Geometry check sheet. Reference: the model listing, model coordinates, mm. Face numbers are marked on the shaded views. Coordinates: 2 decimals unless noted, no trailing zeros. Loops run counter-clockwise (first coordinate to the right, second up) from the corner with the lowest first, then second, coordinate; pieces in that order, holes last.
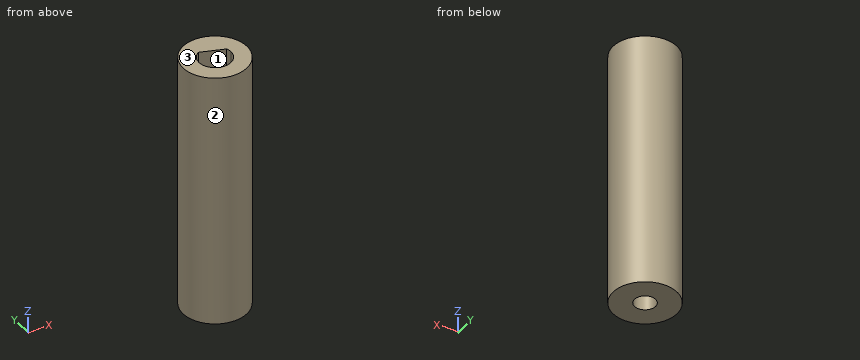
from build123d import *

# Parameters (mm, degrees)
F0_R     = 5
F1_DEPTH = 40
F3_DEPTH = 24
F4_R     = 1.65
F5_DEPTH = 25.4


with BuildPart() as f1:
    # F0 (on Top) → F1 (new body)
    with BuildSketch(Plane.XY):
        Circle(F0_R)
    extrude(amount=F1_DEPTH)

    # F2 (on face) → F3 (cut)
    with BuildSketch(Plane.XY.offset(40)):
        with BuildLine():
            ThreePointArc((-1.309686, 2.129489), (-1.219792, -2.182225), (2.5, 0))
            ThreePointArc((2.5, 0), (2.464167, 0.421758), (2.357696, 0.831425))
            Line((2.357696, 0.831425), (-1.309686, 2.129489))
        make_face()
    extrude(amount=-F3_DEPTH, mode=Mode.SUBTRACT)

    # F4 (on face) → F5 (cut)
    with BuildSketch(Plane(origin=(0, 0, 0), x_dir=(1, 0, 0), z_dir=(0, 0, -1))):
        Circle(F4_R)
    extrude(amount=-F5_DEPTH, mode=Mode.SUBTRACT)


solid = f1.part
(1) Sectioned sample at B-B on x = -0.75. Record the cut outline in (y, z).
Findings:
outline: (-4.94, 0) - (-1.47, 0) - (-1.47, 16) - (-2.38, 16) - (-2.38, 40) - (-4.94, 40) - close; (1.47, 0) - (4.94, 0) - (4.94, 40) - (1.93, 40) - (1.93, 16) - (1.47, 16) - close
(2) Sectioned sample at D-D on z = 7. Record the cut outline in (x, y), and give its area (3 significant figures).
Findings:
outline: circle Ø10 at (0, 0); hole circle Ø3.3 at (0, 0)
area: 70.0 mm2
(3) Scan lines: L1, parallel to Y at x = 0, z = 15.5; L2, parallel to Z at x = -1.75, y = -1.75; L3, parallel to Y at x = -2, z = 37.5. Record each from-to range of solid material in increasing order.
Findings:
L1: y = -5 to -1.65, 1.65 to 5
L2: z = 0 to 16
L3: y = -4.58 to -1.5, 1.5 to 4.58
(4) Gauge pin test, flat ends, axial feed: pin 1 Ø1.5 at (y, z) = (4, 23) entering from +X; pin 2 Ø4 at (x, z) = (-3, 31.5) entering from +Y. Record the tip position at first contact, or that the pin passes through.
Findings:
pin 1: stops at x = 3.8
pin 2: stops at y = 4.9
(5) Sectioned sample at C-C on x = -3. Record the cut outline in (y, z), and give its area (3 significant figures).
Findings:
outline: (-4, 0) - (4, 0) - (4, 40) - (-4, 40) - close
area: 320 mm2
(6) Sectioned sample at A-A on z = 25. Record the cut outline in (x, y).
Findings:
outline: circle Ø10 at (0, 0); hole (-1.31, 2.13) arc R2.5 ccw (long way) to (2.5, 0) arc R2.5 ccw to (2.36, 0.83) - (1, 1.31) arc R1.65 ccw to (0.05, 1.65) - close
(7) Draft check along Y on the marked faces 1, 2 and 3. Enter one of: +Y half, -Y half, draft (parallel to the pull), parting line (faces both ways), or undercut.
Findings:
face 1: undercut
face 2: parting line
face 3: draft
